Verification items for the finished model (mm, model axes). Give positions to 0.01 mm unless a question says otherwise; leave off trailing zeros. Write each loop counter-clockwise with the first axis right and the second up, starting at its lowest first coordinate (ties: lowest second). Pieces come first, ordered by that corner, then holes. Notation, with made-up numbers: M -5,16.5 L 29,16.5 A22 cw 29,41.5 Z; hole C 71.25,25 d2. An arc over 180 degrees is marked long. Write item = value, one per line.
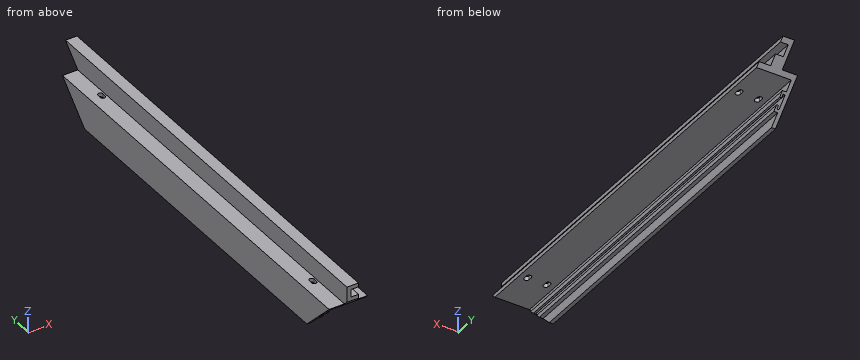
from build123d import *

# Parameters (mm, degrees)
F1_DEPTH = 304.8
F3_DEPTH = 25.4
F5_DEPTH = 50.8
F7_DEPTH = 25.4


with BuildPart() as f1:
    # F0 (on Front) → F1 (new body)
    with BuildSketch(Plane.XZ):
        Polygon((0, 22.86), (0, 0), (2.54, 0), (2.54, 6.35), (5.08, 6.35), (5.08, 9.144), (3.81, 9.144), (3.81, 7.62), (2.54, 7.62), (2.54, 13.97), (3.81, 13.97), (3.81, 12.446), (5.08, 12.446), (5.08, 15.24), (2.54, 15.24), (2.54, 20.32), (25.4, 20.32), (25.4, 22.86), (17.78, 22.86), (17.78, 27.94), (12.7, 27.94), (12.7, 33.02), (17.78, 33.02), (17.78, 35.56), (10.16, 35.56), (10.16, 22.86), align=None)
    extrude(amount=F1_DEPTH)

    # F2 (on face) → F3 (cut)
    with BuildSketch(Plane(origin=(0, 0, 0), x_dir=(0, -1, 0), z_dir=(-1, 0, 0))):
        Polygon((0, 38.1), (0, 0), (38.1, 0), align=None)
        Polygon((304.8, 0), (304.8, 38.1), (266.7, 0), align=None)
    extrude(amount=-F3_DEPTH, mode=Mode.SUBTRACT)

    # F4 (on face) → F5 (cut, symmetric)
    with BuildSketch(Plane.YZ.offset(2.54)):
        Polygon((-292.1, 25.4), (-292.1, 35.56), (-302.26, 35.56), align=None)
    extrude(amount=F5_DEPTH, both=True, mode=Mode.SUBTRACT)

    # F6 (on face) → F7 (cut)
    with BuildSketch(Plane.XY.offset(22.86)):
        with BuildLine():
            ThreePointArc((9.2075, -259.805714), (7.62, -258.218214), (6.0325, -259.805714))
            Line((6.0325, -259.805714), (6.0325, -262.345714))
            ThreePointArc((6.0325, -262.345714), (7.62, -263.933214), (9.2075, -262.345714))
            Line((9.2075, -262.345714), (9.2075, -259.805714))
        make_face()
        with BuildLine():
            Line((21.9075, -262.345714), (21.9075, -259.805714))
            ThreePointArc((21.9075, -259.805714), (20.32, -258.218214), (18.7325, -259.805714))
            Line((18.7325, -259.805714), (18.7325, -262.345714))
            ThreePointArc((18.7325, -262.345714), (20.32, -263.933214), (21.9075, -262.345714))
        make_face()
        with BuildLine():
            Line((9.2075, -44.994286), (9.2075, -42.454286))
            ThreePointArc((9.2075, -42.454286), (7.62, -40.866786), (6.0325, -42.454286))
            Line((6.0325, -42.454286), (6.0325, -44.994286))
            ThreePointArc((6.0325, -44.994286), (7.62, -46.581786), (9.2075, -44.994286))
        make_face()
        with BuildLine():
            ThreePointArc((21.9075, -42.454286), (20.32, -40.866786), (18.7325, -42.454286))
            Line((18.7325, -42.454286), (18.7325, -44.994286))
            ThreePointArc((18.7325, -44.994286), (20.32, -46.581786), (21.9075, -44.994286))
            Line((21.9075, -44.994286), (21.9075, -42.454286))
        make_face()
    extrude(amount=-F7_DEPTH, mode=Mode.SUBTRACT)


solid = f1.part
1) Cross-section at A-A on y = -66. Record the boundary of the cut face in (x, z), plus the area to 3 significant figures.
From the geometry:
outline = M 0,0 L 2.54,0 L 2.54,6.35 L 5.08,6.35 L 5.08,9.14 L 3.81,9.14 L 3.81,7.62 L 2.54,7.62 L 2.54,13.97 L 3.81,13.97 L 3.81,12.45 L 5.08,12.45 L 5.08,15.24 L 2.54,15.24 L 2.54,20.32 L 25.4,20.32 L 25.4,22.86 L 17.78,22.86 L 17.78,27.94 L 12.7,27.94 L 12.7,33.02 L 17.78,33.02 L 17.78,35.56 L 10.16,35.56 L 10.16,22.86 L 0,22.86 Z
area = 197 mm^2
2) Material ranges on probe 1 along Z at (x, y) = (4, -129); probe 2 along Z at (x, y) = (13.5, -202); probe 3 along Y at (x, z) = (19.5, 22), recorded low to high. Write a range as from..to.
From the geometry:
probe_1 = 6.35..9.14, 12.45..15.24, 20.32..22.86
probe_2 = 20.32..27.94, 33.02..35.56
probe_3 = -288.7..-263.71, -258.45..-46.35, -41.09..-16.1
3) Cross-section at B-B on z = 2.5. Record the boundary of the cut face in (x, y), plus the area to 3 significant figures.
From the geometry:
outline = M 0,-269.2 L 2.54,-269.2 L 2.54,-35.6 L 0,-35.6 Z
area = 593 mm^2
4) Depth check by flat-ended pin: P1, Ø3, axis at y = -154, z = 14.5, coming from the +X side; P2, Ø5, axis at x = 5, y = -263, coming from the -Z side; P3, Ø1.3, axis at y = -205.5, z = 34.5, coming from the +X side; P4, Ø1.5, axis at x = 12, y = -77, coming from the -Z side. Enter the tip coordinate at first touch or a pass-through.
From the geometry:
P1 = 5.08
P2 = 0
P3 = 17.78
P4 = 20.32
